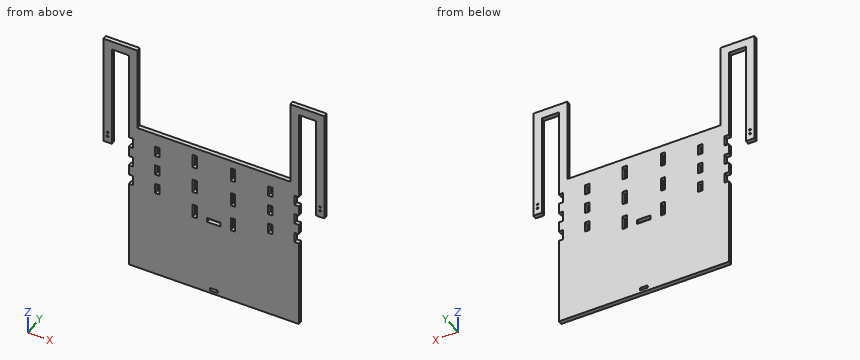
from build123d import *

# Parameters (mm, degrees)
F0_W     = 12.7
F0_H     = 6.35
F0_W_2   = 6.35
F0_H_2   = 77.47
F0_R     = 0.635
F0_W_3   = 3.175
F0_H_3   = 7.62
F0_H_4   = 10.16
F0_W_4   = 10.16
F0_H_5   = 3.175
F1_DEPTH = 3.175


# Not quite as in the source:
# - a feature names something its author has since deleted; it is built from what else it names


with BuildPart() as f1:
    # F0 (on Front) → F1 (new body)
    with BuildSketch(Plane.XZ):
        Polygon((-63.5, 57.15), (-57.15, 57.15), (-57.15, 120.65), (-63.5, 120.65), (-63.5, 114.3), align=None)
        with Locations((-69.85, 117.475)):
            Rectangle(F0_W, F0_H)
        with Locations((-79.375, 117.475)):
            Rectangle(F0_W_2, F0_H)
        with Locations((-79.375, 75.565)):
            Rectangle(F0_W_2, F0_H_2)
        with Locations((-79.375, 41.7701676488)):
            Circle(F0_R, mode=Mode.SUBTRACT)
        with Locations((-79.375, 44.9451676488)):
            Circle(F0_R, mode=Mode.SUBTRACT)
        Polygon((57.15, 57.15), (63.5, 57.15), (63.5, 114.3), (63.5, 120.65), (57.15, 120.65), align=None)
        Polygon((63.5, 120.65), (63.5, 114.3), (76.2, 114.3), (82.55, 114.3), (82.55, 120.65), align=None)
        with Locations((79.375, 75.565)):
            Rectangle(F0_W_2, F0_H_2)
        with Locations((79.375, 41.7701676488)):
            Circle(F0_R, mode=Mode.SUBTRACT)
        with Locations((79.375, 44.9451676488)):
            Circle(F0_R, mode=Mode.SUBTRACT)
        Polygon((63.5, 46.99), (63.5, 57.15), (57.15, 57.15), (-57.15, 57.15), (-63.5, 57.15), (-63.5, 46.99), (-60.325, 46.99), (-60.325, 39.37), (-63.5, 39.37), (-63.5, 31.75), (-60.325, 31.75), (-60.325, 24.13), (-63.5, 24.13), (-63.5, 16.51), (-60.325, 16.51), (-60.325, 8.89), (-63.5, 8.89), (-63.5, -57.15), (63.5, -57.15), (63.5, 8.89), (60.325, 8.89), (60.325, 16.51), (63.5, 16.51), (63.5, 24.13), (60.325, 24.13), (60.325, 31.75), (63.5, 31.75), (63.5, 39.37), (60.325, 39.37), (60.325, 46.99), align=None)
        with Locations((-42.2275, 12.7)):
            Rectangle(F0_W_3, F0_H_3, mode=Mode.SUBTRACT)
        with Locations((-42.2275, 27.94)):
            Rectangle(F0_W_3, F0_H_3, mode=Mode.SUBTRACT)
        with Locations((-14.2875, 5.3341257808)):
            Rectangle(F0_W_3, F0_H_4, mode=Mode.SUBTRACT)
        with Locations((-14.2875, 25.6541257808)):
            Rectangle(F0_W_3, F0_H_4, mode=Mode.SUBTRACT)
        with BuildLine():
            ThreePointArc((2.8175964356, -53.0858742192), (2.9972, -54.1078126547), (2.8175964356, -55.1297510902))
            Line((2.8175964356, -55.1297510902), (-2.8175964356, -55.1297510902))
            ThreePointArc((-2.8175964356, -55.1297510902), (-2.9972, -54.1078126547), (-2.8175964356, -53.0858742192))
            Line((-2.8175964356, -53.0858742192), (2.8175964356, -53.0858742192))
        make_face(mode=Mode.SUBTRACT)
        with Locations((0, 1.8416257808)):
            Rectangle(F0_W_4, F0_H_5, mode=Mode.SUBTRACT)
        with Locations((14.2875, 5.3341257808)):
            Rectangle(F0_W_3, F0_H_4, mode=Mode.SUBTRACT)
        with Locations((14.2875, 25.6541257808)):
            Rectangle(F0_W_3, F0_H_4, mode=Mode.SUBTRACT)
        with Locations((42.2275, 12.7)):
            Rectangle(F0_W_3, F0_H_3, mode=Mode.SUBTRACT)
        with Locations((42.2275, 27.94)):
            Rectangle(F0_W_3, F0_H_3, mode=Mode.SUBTRACT)
        with Locations((-42.2275, 43.18)):
            Rectangle(F0_W_3, F0_H_3, mode=Mode.SUBTRACT)
        with Locations((-14.2875, 45.9741257808)):
            Rectangle(F0_W_3, F0_H_4, mode=Mode.SUBTRACT)
        with Locations((14.2875, 45.9741257808)):
            Rectangle(F0_W_3, F0_H_4, mode=Mode.SUBTRACT)
        with Locations((42.2275, 43.18)):
            Rectangle(F0_W_3, F0_H_3, mode=Mode.SUBTRACT)
    extrude(amount=F1_DEPTH)


solid = f1.part
Model file for the job. Use its own axes, mm. Give positions to 0.01 mm unless a question says otherwise; leave off trailing zeros. Loops run counter-clockwise (first coordinate to the right, second up) from the corner with the lowest first, then second, coordinate; pieces in that order, holes last.
Item 1: Slice it at D-D (y = -1.4). Give the number of separate pieces and of enclosed holes in the cut face, plus the area to 3 significant figures.
Check values:
separate pieces: 1
enclosed holes: 18
area: 16,000 mm2
Item 2: Slice it at B-B (x = 66.5). Write the cut outline in (y, z) (3 decimals).
Check values:
outline: (-3.175, 114.3) - (0, 114.3) - (0, 120.65) - (-3.175, 120.65) - close
Item 3: Slice it at A-A (z = 92.5). Write the cut outline in (x, y) (3 decimals).
Check values:
outline: (-82.55, -3.175) - (-76.2, -3.175) - (-76.2, 0) - (-82.55, 0) - close; (-63.5, -3.175) - (-57.15, -3.175) - (-57.15, 0) - (-63.5, 0) - close; (57.15, -3.175) - (63.5, -3.175) - (63.5, 0) - (57.15, 0) - close; (76.2, -3.175) - (82.55, -3.175) - (82.55, 0) - (76.2, 0) - close
Item 4: Drop flat-ended pins along their axis: P1, Ø1, axis at y = -2.5, z = -26, coming from the +X side; P2, Ø1.5, axis at y = -0.5, z = -13.5, coming from the -X side; P3, Ø1, axis at y = -1.5, z = 11, coming from the +X side (3 decimals). Give the stop position or say it passes through.
Check values:
P1: stops at x = 63.5
P2: stops at x = -63.5
P3: stops at x = 60.325
Item 5: Drill centre lines: line 1 along Z through (x, y) = (-15, -3); line 2 along X through (y, z) = (-1.6, 7) (3 decimals); line 3 along X through (y, z) = (-1, 93.5). Where is each one in solid material? Low to high.
Check values:
line 1: z = -57.15 to 0.25, 10.41 to 20.57, 30.73 to 40.89, 51.05 to 57.15
line 2: x = -63.5 to -15.875, -12.7 to 12.7, 15.875 to 63.5
line 3: x = -82.55 to -76.2, -63.5 to -57.15, 57.15 to 63.5, 76.2 to 82.55
Item 6: Slice it at C-C (z = -45.5). Write the cut outline in (x, y) (3 decimals).
Check values:
outline: (-63.5, -3.175) - (63.5, -3.175) - (63.5, 0) - (-63.5, 0) - close
